Work out the finished part from the listing and answer in its coordinate system (mm). A direction names the side the tool comes from. Round coordinates to 2 decimals unless told otherwise and drop trailing zeros. Write each loop counter-clockwise with the first axis right and the second up, starting at its lowest first coordinate (ties: lowest second). Pieces come first, ordered by that corner, then holes. Notation, with made-up numbers: M 22,-23.75 L 54,-23.75 A19 ccw 54,-1.75 Z; hole C 8.25,-6.75 d11. An arc over 180 degrees is marked long. One line per item, written item: value. Start each with the question number.
Q1. Consider probe 1 along X at (y, z) = (1.95, -4.25); probe 2 along Z at (x, y) = (20.75, 3); probe 3 along X at (y, z) = (3.05, -15.75). Determine where each line is inside the solid, lowest interval first.
Q2. The mould has two halves that part along Z. Classify faces 3 (the cylindrical face through (12.8, 2.5, -12.1)), 4 (the flat face through (15, 2, -20)), 5 (the flat face through (15, 2, 0)), 6 (the flat face through (15, 0, -12)): released by +Z, released by -Z, zero draft, split by the parting line, or undercut.
Q3. A tool of negligible diameter and unlimited length cuts with its end or side. For faces 1 (the flat face through (6, 3, -6.038)), 2 (the flat face through (30, 2, -10)), from which of +Z, -Z, +X, -X, +Y, -Y can it reach the whole face along a straight path? Write none if from no direction.
Q4. Find section C-C (z = -4.75). Write down the section's boundary in (x, y).
Q5. Find section A-A (z = -10). Write down the section's boundary in (x, y), and give its area (3 significant figures).
Q6. Find section B-B (y = 1.25). Count the separate pieces of the cut face and the enclosed holes in it, and give its area (3 significant figures).
from build123d import *

# Parameters (mm, degrees)
SKETCH2_W           = 30
SKETCH2_H           = 20
BOSS_EXTRUDE1_DEPTH = 5
SKETCH5_R           = 1.35
SKETCH5_R_2         = 1.6
SKETCH5_R_3         = 2.1
SKETCH5_R_4         = 1.55
SKETCH5_R_5         = 1.3
SKETCH5_R_6         = 2.05
SKETCH5_R_7         = 1.65
SKETCH5_R_8         = 2.15
CUT_EXTRUDE3_DEPTH  = 37.400549446


with BuildPart() as part:
    # Sketch2 → Boss-Extrude1 (new body)
    with BuildSketch(Plane(origin=(0, 0, 0), x_dir=(1, 0, 0), z_dir=(0, 1, 0))):
        with Locations((15, 10)):
            Rectangle(SKETCH2_W, SKETCH2_H)
    extrude(amount=BOSS_EXTRUDE1_DEPTH)

    # Sketch5 → Cut-Extrude3 (cut, through all)
    with BuildSketch(Plane(origin=(0, 5, 0), x_dir=(1, 0, 0), z_dir=(0, 1, 0))):
        with Locations(Location((27.444530449, 10, 0), (0, 0, 270))):
            Circle(SKETCH5_R)
        with Locations(Location((20.700795765, 10, 0), (0, 0, 270))):
            Circle(SKETCH5_R_2)
        with Locations(Location((12.732583582, 10, 0), (0, 0, 270))):
            Circle(SKETCH5_R_3)
        with Locations(Location((20.700795765, 16.093784601, 0), (0, 0, 270))):
            Circle(SKETCH5_R_4)
        with Locations(Location((27.444530449, 16.093784601, 0), (0, 0, 270))):
            Circle(SKETCH5_R_5)
        with Locations(Location((12.732583582, 16.093784601, 0), (0, 0, 270))):
            Circle(SKETCH5_R_6)
        with Locations(Location((20.700795765, 4.387736866, 0), (0, 0, 270))):
            Circle(SKETCH5_R_7)
        with Locations(Location((27.444530449, 4.387736866, 0), (0, 0, 270))):
            Circle(SKETCH5_R_5)
        with Locations(Location((12.732583582, 4.387736866, 0), (0, 0, 270))):
            Circle(SKETCH5_R_8)
        with BuildLine():
            Line((4.365184557, 11.6), (7.085478659, 11.6))
            ThreePointArc((7.085478659, 11.6), (5.725331608, 7.9), (4.365184557, 11.6))
        make_face()
        with BuildLine():
            Line((4.346926733, 6.037736866), (7.103736483, 6.037736866))
            ThreePointArc((7.103736483, 6.037736866), (5.725331608, 2.237736866), (4.346926733, 6.037736866))
        make_face()
        with BuildLine():
            Line((4.383690822, 17.643784601), (7.066972395, 17.643784601))
            ThreePointArc((7.066972395, 17.643784601), (5.725331608, 14.043784601), (4.383690822, 17.643784601))
        make_face()
    extrude(amount=-CUT_EXTRUDE3_DEPTH, mode=Mode.SUBTRACT)


solid = part.part
The answers:
1. probe 1: 0 to 3.58, 7.87 to 10.59, 14.88 to 19.06, 22.35 to 26.15, 28.74 to 30
1. probe 2: -20 to -17.64, -14.54 to -11.6, -8.4 to -6.04, -2.74 to 0
1. probe 3: 0 to 3.7, 7.75 to 10.71, 14.75 to 19.19, 22.21 to 26.19, 28.7 to 30
2. face 3: undercut
2. face 4: released by -Z
2. face 5: released by +Z
2. face 6: zero draft
3. face 1: +Y, -Y
3. face 2: +Z, -Z, +X, +Y, -Y
4. outline: M 0,0 L 3.61,0 L 3.61,5 L 0,5 Z; M 7.84,0 L 10.61,0 L 10.61,5 L 7.84,5 Z; M 14.85,0 L 19.09,0 L 19.09,5 L 14.85,5 Z; M 22.31,0 L 26.2,0 L 26.2,5 L 22.31,5 Z; M 28.69,0 L 30,0 L 30,5 L 28.69,5 Z
5. outline: M 0,0 L 3.63,0 L 3.63,5 L 0,5 Z; M 7.83,0 L 10.63,0 L 10.63,5 L 7.83,5 Z; M 14.83,0 L 19.1,0 L 19.1,5 L 14.83,5 Z; M 22.3,0 L 26.09,0 L 26.09,5 L 22.3,5 Z; M 28.79,0 L 30,0 L 30,5 L 28.79,5 Z
5. area: 78.5 mm2
6. separate pieces: 1
6. enclosed holes: 12
6. area: 479 mm2
